For this review, take the finished solid that the model builds, in its own axes (mm). A direction names the side the tool comes from. Round coordinates to 2 decimals unless told otherwise and drop trailing zeros. Write each loop counter-clockwise with the first axis right and the second up, starting at its lowest first coordinate (ties: lowest second). Pieces come first, ordered by that corner, then holes. Notation, with made-up numbers: (77.25, 3.5) - (111.25, 3.5) arc R10 ccw to (111.25, 10.5) - close; hole circle Ø1 at (-23.5, 45). An arc over 180 degrees is marked (long way). One line per item, written item: value. Start each with the question number.
Q1. For probe 1 along Z at (x, y) = (7.75, 1.75); probe 2 along Y at (x, z) = (5.5, -2); probe 3 along X at (y, z) = (-3, 0.25), list the stretches that pass through material, from the lowest coordinate up.
Q2. Add section A-A on x = 6.5. Write out the cut boundary in (y, z), and give its area (3 significant figures).
Q3. Clearance check with flat-ended pins moving along their axes: pin 1 Ø2 at (x, y) = (3, 1.5) entering from +Z; pin 2 Ø1 at (x, z) = (8, -0.5) entering from -Y; pin 3 Ø4 at (y, z) = (1, 3) entering from +X. State where each tip first meets the part, or that it passes through.
Q4. Tool access review of faces 1 (the face through (3.451, -1.341, -3.233)), 2 (the face through (10, 0, 0)): name each direction out of +Z, -Z, +X, -X, +Y, -Y from which nothing blocks a thin tool from reaching the whole face with its end or side.
```python
from build123d import *

# Parameters (mm, degrees)
CROQUIS1_R              = 3.5
SALIENTE_EXTRUIR1_DEPTH = 10
REDONDEO1_R             = 3
CROQUIS2_R              = 3.55
SALIENTE_EXTRUIR2_DEPTH = 0.5


with BuildPart() as part:
    # Croquis1 → Saliente-Extruir1 (new body)
    with BuildSketch(Plane(origin=(0, 0, 0), x_dir=(0, 0, -1), z_dir=(1, 0, 0))):
        Circle(CROQUIS1_R)
    extrude(amount=SALIENTE_EXTRUIR1_DEPTH)

    # Redondeo1
    redondeo1_edges = [part.edges().sort_by_distance(p)[0] for p in [
        (10, 0, 3.5),
    ]]
    fillet(redondeo1_edges, radius=REDONDEO1_R)

    # Croquis2 → Saliente-Extruir2 (add)
    with BuildSketch(Plane.ZY):
        Circle(CROQUIS2_R)
    extrude(amount=SALIENTE_EXTRUIR2_DEPTH)


solid = part.part
```
Result set:
1. probe 1: z = -2.92 to 2.92
1. probe 2: y = -2.87 to 2.87
1. probe 3: x = -0.5 to 8.64
2. outline: circle Ø7 at (0, 0)
2. area: 38.5 mm^2
3. pin 1: stops at z = 3.46
3. pin 2: stops at y = -3.44
3. pin 3: stops at x = 9.93
4. face 1: +X
4. face 2: +Z, -Z, +X, +Y, -Y
